Read the model definition and answer for the solid it produces. Units are mm, in the model's axes. A direction names the side the tool comes from. Round coordinates to 2 decimals unless told otherwise and drop trailing zeros. Write each loop counter-clockwise with the first axis right and the second up, starting at its lowest first coordinate (ties: lowest second). Pieces come first, ordered by that corner, then holes. Notation, with made-up numbers: (76, 57) - (95, 57) arc R33 ccw to (95, 86) - close; hole circle Ø4 at (-26, -1.75). An arc over 180 degrees is marked (long way). Answer as CSV lines item,"result". Start each with the question number.
1) Each of these flat-tipped pins is pushed along its axis until it touches: pin 1 (3 mm diameter, centred on y = 32.5, z = 4.5, fed in from -X); pin 2 (1.9 mm diameter, centred on y = -28.5, z = 4.5, fed in from +X); pin 3 (3 mm diameter, centred on x = 24, z = 2, fed in from +Y). Where does it stop, or does it pass through?
2) Consider line 1 along X through (y, z) = (14, 2.5); line 2 along Y through (x, z) = (-29, 4); line 3 along X through (y, z) = (-29, 3.5). Determine where each line is inside the solid, lowest interval first.
3) Find section B-B on y = 24.5. Determine the outline of the cut face in (x, z).
4) Which of the six approach directions +Z, -Z, +X, -X, +Y, -Y give full straight-line access (tool end or side, diameter ignored) to faces 1 (the flat face through (41.341, -3, 3)), 2 (the flat face through (-27, 8.296, 3)), 3 (the flat face through (11.289, -31, 3)), 4 (the flat face through (2, 22, 0)), 5 (the flat face through (-24, -13.358, 3))?
5) Find section A-A on z = 1.5. Determine the outline of the cut face in (x, y).
6) Find section C-C on x = 22. Determine the outline of the cut face in (y, z), then the cut area to 3 significant figures.
7) For a pull along Y with two mould halves and no side action, classify faces 6 (the flat face through (-9.15, 78.67, 3.13)), 7 (the flat face through (-36.279, -2, 3)), 8 (the flat face through (2, -43.45, 3)), 9 (the cylindrical face through (14.443, -16.882, 3.131)) as +Y half, -Y half, draft (parallel to the pull), parting line (faces both ways), or undercut.
from build123d import *

# Parameters (mm, degrees)
F1_DEPTH = 6.35


with BuildPart() as f1:
    # F0 (on Top) → F1 (new body)
    with BuildSketch(Plane.XY):
        with BuildLine():
            Line((11.2930470291, 11.6638336243), (11.2889658673, 8.2962913439))
            Line((11.2889658673, 8.2962913439), (12.0783096254, 8.2962913439))
            ThreePointArc((12.0783096254, 8.2962913439), (11.597122228, 9.9594124709), (11.2930470291, 11.6638336243))
        make_face()
        with BuildLine():
            ThreePointArc((37.3601643932, 8.2962913439), (38.2870822741, 3.6378996321), (41.3408465683, 0))
            Line((41.3408465683, 0), (41.3408465683, 8.2962913439))
            Line((41.3408465683, 8.2962913439), (37.3601643932, 8.2962913439))
        make_face()
        Polygon((-2.8123026714, 44.2937612534), (-2.8123026714, 8.2962913439), (4.7809146345, 8.2962913439), (4.2298541355, 62.0834718136), (0, 65.1047974825), (-2.8123026714, 61.1675754189), (-2.8123026714, 51.8869794905), align=None)
        with BuildLine():
            Line((-10.813491419, 44.2937612534), (-10.8399443516, 12.7670755447))
            ThreePointArc((-10.8399443516, 12.7670755447), (-7.807634986, 11.5598221537), (-7.8491980914, 8.2962913439))
            Line((-7.8491980914, 8.2962913439), (-2.8123026714, 8.2962913439))
            Line((-2.8123026714, 8.2962913439), (-2.8123026714, 44.2937612534))
            Line((-2.8123026714, 44.2937612534), (-2.8123026714, 51.8869794905))
            Line((-2.8123026714, 51.8869794905), (-2.8123026714, 61.1675754189))
            Line((-2.8123026714, 61.1675754189), (0, 65.1047974825))
            Line((0, 65.1047974825), (4.2298541355, 62.0834718136))
            Line((4.2298541355, 62.0834718136), (4.7809146345, 8.2962913439))
            Line((4.7809146345, 8.2962913439), (7.9583702463, 8.2962913439))
            ThreePointArc((7.9583702463, 8.2962913439), (8.7402628967, 10.8568667256), (11.2930470291, 11.6638336243))
            Line((11.2930470291, 11.6638336243), (11.3227786668, 36.1966877298))
            Line((11.3227786668, 36.1966877298), (11.3565914662, 64.0970841157))
            Line((11.3565914662, 64.0970841157), (0, 76.3540118933))
            Line((0, 76.3540118933), (-10.813491419, 66.3348287344))
            Line((-10.813491419, 66.3348287344), (-10.813491419, 44.2937612534))
        make_face()
        with BuildLine():
            Line((-7.8520236744, -16.7259749874), (-7.8491980914, -13.3584365249))
            Line((-7.8491980914, -13.3584365249), (-12.0928995311, -13.3584365249))
            ThreePointArc((-12.0928995311, -13.3584365249), (-10.8775211038, -16.1819833799), (-7.8520236744, -16.7259749874))
        make_face()
        with BuildLine():
            ThreePointArc((11.2889658673, -38.08565063), (8.4977328176, -40.3265486279), (6.7495256662, -43.4500686824))
            Line((6.7495256662, -43.4500686824), (11.2889658673, -43.4500686824))
            Line((11.2889658673, -43.4500686824), (11.2889658673, -38.08565063))
        make_face()
        with BuildLine():
            Line((11.2889658673, -13.3584365249), (11.2889658673, -18.7083456713))
            ThreePointArc((11.2889658673, -18.7083456713), (14.4627701422, -16.8299590512), (13.2178198546, -13.3584365249))
            Line((13.2178198546, -13.3584365249), (11.2889658673, -13.3584365249))
        make_face()
        with BuildLine():
            ThreePointArc((41.3408465683, -8.0150617286), (38.6442879923, -10.0493741157), (37.9660837352, -13.3584365249))
            Line((37.9660837352, -13.3584365249), (41.3408465683, -13.3584365249))
            Line((41.3408465683, -13.3584365249), (41.3408465683, -8.0150617286))
        make_face()
        with BuildLine():
            Line((-10.8399443516, 12.7670755447), (-10.8436956293, 8.2962913439))
            Line((-10.8436956293, 8.2962913439), (-10.813491419, 8.2962913439))
            Line((-10.813491419, 8.2962913439), (-7.8491980914, 8.2962913439))
            ThreePointArc((-7.8491980914, 8.2962913439), (-7.807634986, 11.5598221537), (-10.8399443516, 12.7670755447))
        make_face()
        with BuildLine():
            ThreePointArc((-5.6246044114, -43.4500686824), (-5.6592907147, -40.9529633104), (-7.8713791675, -39.793910656))
            Line((-7.8713791675, -39.793910656), (-7.8744469211, -43.4500686824))
            Line((-7.8744469211, -43.4500686824), (-5.6246044114, -43.4500686824))
        make_face()
        with BuildLine():
            ThreePointArc((11.2930470291, 11.6638336243), (8.7402628967, 10.8568667256), (7.9583702463, 8.2962913439))
            Line((7.9583702463, 8.2962913439), (11.2889658673, 8.2962913439))
            Line((11.2889658673, 8.2962913439), (11.2930470291, 11.6638336243))
        make_face()
        with BuildLine():
            Line((-12.0928995311, -13.3584365249), (-7.8491980914, -13.3584365249))
            Line((-7.8491980914, -13.3584365249), (-7.8520236744, -16.7259749874))
            Line((-7.8520236744, -16.7259749874), (-7.8713791675, -39.793910656))
            ThreePointArc((-7.8713791675, -39.793910656), (-5.6592907147, -40.9529633104), (-5.6246044114, -43.4500686824))
            Line((-5.6246044114, -43.4500686824), (6.7495256662, -43.4500686824))
            ThreePointArc((6.7495256662, -43.4500686824), (8.4977328176, -40.3265486279), (11.2889658673, -38.08565063))
            Line((11.2889658673, -38.08565063), (11.2889658673, -18.7083456713))
            Line((11.2889658673, -18.7083456713), (11.2889658673, -13.3584365249))
            Line((11.2889658673, -13.3584365249), (13.2178198546, -13.3584365249))
            Line((13.2178198546, -13.3584365249), (37.9660837352, -13.3584365249))
            ThreePointArc((37.9660837352, -13.3584365249), (38.6442879923, -10.0493741157), (41.3408465683, -8.0150617286))
            Line((41.3408465683, -8.0150617286), (41.3408465683, 0))
            ThreePointArc((41.3408465683, 0), (38.2870822741, 3.6378996321), (37.3601643932, 8.2962913439))
            Line((37.3601643932, 8.2962913439), (31.7790135741, 8.2962913439))
            Line((31.7790135741, 8.2962913439), (17.8106164583, 8.2962913439))
            Line((17.8106164583, 8.2962913439), (16.0766797152, 8.2962913439))
            Line((16.0766797152, 8.2962913439), (14.3427429721, 8.2962913439))
            Line((14.3427429721, 8.2962913439), (12.0783096254, 8.2962913439))
            Line((12.0783096254, 8.2962913439), (11.2889658673, 8.2962913439))
            Line((11.2889658673, 8.2962913439), (7.9583702463, 8.2962913439))
            Line((7.9583702463, 8.2962913439), (4.7809146345, 8.2962913439))
            Line((4.7809146345, 8.2962913439), (-2.8123026714, 8.2962913439))
            Line((-2.8123026714, 8.2962913439), (-7.8491980914, 8.2962913439))
            Line((-7.8491980914, 8.2962913439), (-10.813491419, 8.2962913439))
            Line((-10.813491419, 8.2962913439), (-10.8436956293, 8.2962913439))
            Line((-10.8436956293, 8.2962913439), (-18.5611955822, 8.2962913439))
            Line((-18.5611955822, 8.2962913439), (-27.1387170069, 8.2962913439))
            Line((-27.1387170069, 8.2962913439), (-31.7087078001, 8.2962913439))
            ThreePointArc((-31.7087078001, 8.2962913439), (-32.9074253056, 5.0668217141), (-36.2786985934, 4.3590688147))
            Line((-36.2786985934, 4.3590688147), (-36.2786985934, -8.5775218904))
            ThreePointArc((-36.2786985934, -8.5775218904), (-33.5801197144, -10.4479621169), (-32.0602469146, -13.3584365249))
            Line((-32.0602469146, -13.3584365249), (-12.0928995311, -13.3584365249))
        make_face()
        with BuildLine():
            Line((-18.5611955822, 15.7010573894), (-18.5611955822, 8.2962913439))
            Line((-18.5611955822, 8.2962913439), (-10.8436956293, 8.2962913439))
            Line((-10.8436956293, 8.2962913439), (-10.8399443516, 12.7670755447))
            Line((-10.8399443516, 12.7670755447), (-10.813491419, 44.2937612534))
            Line((-10.813491419, 44.2937612534), (-10.813491419, 66.3348287344))
            Line((-10.813491419, 66.3348287344), (0, 76.3540118933))
            Line((0, 76.3540118933), (11.3565914662, 64.0970841157))
            Line((11.3565914662, 64.0970841157), (11.3227786668, 36.1966877298))
            Line((11.3227786668, 36.1966877298), (11.2930470291, 11.6638336243))
            ThreePointArc((11.2930470291, 11.6638336243), (11.597122228, 9.9594124709), (12.0783096254, 8.2962913439))
            Line((12.0783096254, 8.2962913439), (14.3427429721, 8.2962913439))
            Line((14.3427429721, 8.2962913439), (16.0766797152, 8.2962913439))
            Line((16.0766797152, 8.2962913439), (16.3020100445, 70.7799866796))
            Line((16.3020100445, 70.7799866796), (0, 86.3380655646))
            Line((0, 86.3380655646), (-18.5611955822, 70.7799866796))
            Line((-18.5611955822, 70.7799866796), (-18.5611955822, 15.7010573894))
        make_face()
        with BuildLine():
            Line((-36.2786985934, 8.2962913439), (-36.2786985934, 4.3590688147))
            ThreePointArc((-36.2786985934, 4.3590688147), (-32.9074253056, 5.0668217141), (-31.7087078001, 8.2962913439))
            Line((-31.7087078001, 8.2962913439), (-36.2786985934, 8.2962913439))
        make_face()
        with BuildLine():
            Line((-36.2786985934, -13.3584365249), (-32.0602469146, -13.3584365249))
            ThreePointArc((-32.0602469146, -13.3584365249), (-33.5801197144, -10.4479621169), (-36.2786985934, -8.5775218904))
            Line((-36.2786985934, -8.5775218904), (-36.2786985934, -13.3584365249))
        make_face()
    extrude(amount=F1_DEPTH)


solid = f1.part
Check values:
1,pin 1,"stops at x = -18.56"
1,pin 2,"stops at x = 11.29"
1,pin 3,"stops at y = 8.3"
2,line 1,"x = -18.56 to 16.1"
2,line 2,"y = -13.36 to 8.3"
2,line 3,"x = -7.86 to 11.29"
3,outline,"(-18.56, 0) - (16.14, 0) - (16.14, 6.35) - (-18.56, 6.35) - close"
4,face 1,"+Z, -Z, +X, +Y, -Y"
4,face 2,"+Z, -Z, -X, +Y"
4,face 3,"+Z, -Z, +X, -Y"
4,face 4,"-Z, +X, -X, +Y, -Y"
4,face 5,"+Z, -Z, -X, -Y"
5,outline,"(-36.28, -13.36) - (-12.09, -13.36) arc R3.25 ccw to (-7.85, -16.73) - (-7.87, -43.45) - (11.29, -43.45) - (11.29, -18.71) arc R2.9 ccw to (13.22, -13.36) - (41.34, -13.36) - (41.34, 8.3) - (16.08, 8.3) - (16.3, 70.78) - (0, 86.34) - (-18.56, 70.78) - (-18.56, 8.3) - (-36.28, 8.3) - close"
6,outline,"(-13.36, 0) - (8.3, 0) - (8.3, 6.35) - (-13.36, 6.35) - close"
6,area,"138 mm^2"
7,face 6,"+Y half"
7,face 7,"draft"
7,face 8,"-Y half"
7,face 9,"undercut"
